```python
from build123d import *

# Parameters (mm, degrees)
SKETCH1_W           = 38
SKETCH1_H           = 38
BOSS_EXTRUDE1_DEPTH = 250
FILLET1_R           = 5
SHELL1_T            = -3


with BuildPart() as part:
    # Sketch1 → Boss-Extrude1 (new, symmetric)
    with BuildSketch(Plane(origin=(0, 0, 0), x_dir=(1, 0, 0), z_dir=(0, 1, 0))):
        Rectangle(SKETCH1_W, SKETCH1_H)
    extrude(amount=BOSS_EXTRUDE1_DEPTH, both=True)

    # Fillet1
    fillet1_edges = [part.edges().sort_by_distance(p)[0] for p in [
        (19, 0, 19),
        (-19, 0, 19),
        (-19, 0, -19),
        (19, 0, -19),
    ]]
    fillet(fillet1_edges, radius=FILLET1_R)

    # Shell1
    shell1_openings = [part.faces().sort_by_distance(p)[0] for p in [
        (0, 250, 0),
        (0, -250, 0),
    ]]
    offset(amount=SHELL1_T, openings=shell1_openings, kind=Kind.INTERSECTION)


solid = part.part
```
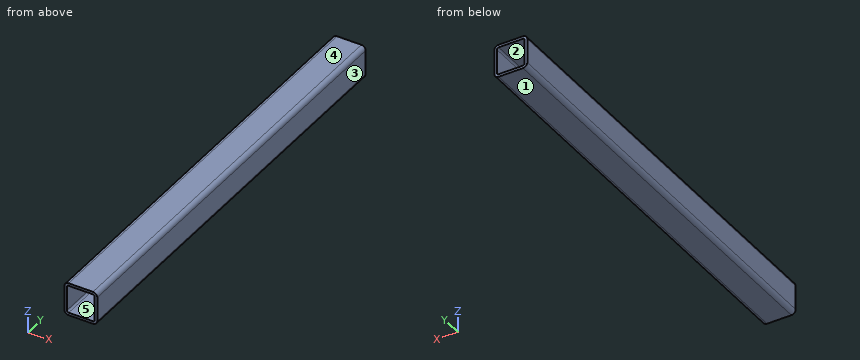
Can you work these out from the model? Positions are in its coordinate system, mm. Face numbers are marked on the shaded views. A direction names the side the tool comes from. Coordinates: 2 decimals unless noted, no trailing zeros. Loops run counter-clockwise (first coordinate to the right, second up) from the corner with the lowest first, then second, coordinate; pieces in that order, holes last. Notation, with made-up numbers: (19.25, 77.25) - (25.25, 77.25) arc R27 ccw to (25.25, 104.25) - close; hole circle Ø1 at (46.25, -4). An arc over 180 degrees is marked (long way). Answer as CSV lines item,"result". Start each with the question number.
1) Which directions (+Z, -Z, +X, -X, +Y, -Y) give clear straight access to the entire face, cutting with the end or side of a thin tool? Please do the marked faces 1 and 2.
2) Thinking about a two-plate mould opening in X: for the marked faces 3, 4 and 5, which applies, pulls with the +X half, pulls with the -X half, needs draft (parallel to the pull), parting line crosses it, or undercut?
3) For pin 1 (2 mm diameter, centred on x = 3.5, z = 14.5, fed in from +Y), with a flat end and sliding along its axis, tell me the tip position at first contact or that it passes through.
4) I need wall thicknesses on line 1 (Z direction, x = -11, y = 142.5); line 2 (Z direction, x = 17.5, y = 95.5). Which ranges of each line are inside material? Lowest first, please. Write a range as from..to.
5) Suppose I cut it at B-B (x = 0). Please give me the cut outline in (y, z).
6) Suppose I cut it at A-A (z = 6.5). Please give me the cut outline in (x, y), plus the area to 3 significant figures.
7) Suppose I cut it at C-C (y = 104). Please give me the cut outline in (x, z).
Check result:
1,face 1,"-Z, +X, -X, +Y, -Y"
1,face 2,"+Y, -Y"
2,face 3,"pulls with the +X half"
2,face 4,"needs draft"
2,face 5,"undercut"
3,pin 1,"passes through"
4,line 1,"z = -19..-16, 16..19"
4,line 2,"z = -17.57..17.57"
5,outline,"(-250, -19) - (250, -19) - (250, -16) - (-250, -16) - close; (-250, 16) - (250, 16) - (250, 19) - (-250, 19) - close"
6,outline,"(-19, -250) - (-16, -250) - (-16, 250) - (-19, 250) - close; (16, -250) - (19, -250) - (19, 250) - (16, 250) - close"
6,area,"3,000 mm²"
7,outline,"(-19, -14) arc R5 ccw to (-14, -19) - (14, -19) arc R5 ccw to (19, -14) - (19, 14) arc R5 ccw to (14, 19) - (-14, 19) arc R5 ccw to (-19, 14) - close; hole (-16, -14) arc R2 ccw to (-14, -16) - (14, -16) arc R2 ccw to (16, -14) - (16, 14) arc R2 ccw to (14, 16) - (-14, 16) arc R2 ccw to (-16, 14) - close"
